Check sheet for the modelled part. Datum: model origin and axes. Units: mm. Give positions to 0.01 mm unless a question says otherwise; leave off trailing zeros. Loops run counter-clockwise (first coordinate to the right, second up) from the corner with the lowest first, then second, coordinate; pieces in that order, holes last. Notation, with made-up numbers: (18.25, -3.75) -> (58.25, -3.75) arc R20 ccw to (58.25, 32.25) -> close; hole circle Ø7 at (65, -7.5). An arc over 180 degrees is marked (long way). Answer as CSV lines item,"result". Start each with the question number.
(1) Section check D-D on z = 2. Enter the section's corners in (x, y), plus the area to 3 significant figures.
(2) Section check B-B on z = 0. Enter the section's corners in (x, y), plus the area to 3 significant figures.
(3) Section check A-A on x = 0. Enter the section's corners in (y, z), plus the area to 3 significant figures.
(4) Material ranges on line 1 (Y direction, x = 0, z = -0.15); line 2 (X direction, y = 14.5, z = 0.45); line 3 (X direction, y = 14.5, z = 0.8), recorded low to high. Write a range as from..to.
(5) Section check C-C on y = 11.75. Enter the section's corners in (x, z).
(6) Release check for a two-part mould opening along X. For faces 1 (the face through (2.385, 9.86, -0.751)), 2 (the face through (-0.098, 15.244, 0.035)), 3 (the face through (0, 0, 0)) record: pulls with the +X half, pulls with the -X half, needs draft (parallel to the pull), parting line crosses it, or undercut.
(7) Gauge pin test, flat ends, axial feed: pin 1 Ø1.5 at (y, z) = (9.5, 1) entering from -X; pin 2 Ø1 at (y, z) = (11.5, -1) entering from -X. Record the tip position at first contact, or that the pin passes through.
from build123d import *

# Parameters (mm, degrees)
CROQUIS1_R                        = 2.5
SALIENTE_EXTRUIR1_DEPTH           = 20
CORTAR_EXTRUIR1_REACH             = 4.5
CROQUIS2_R                        = 0.75
CORTAR_EXTRUIR1_DIRECTION_2_REACH = 4.5


with BuildPart() as part:
    # Croquis1 → Saliente-Extruir1 (new body)
    with BuildSketch(Plane(origin=(0, 0, 0), x_dir=(1, 0, 0), z_dir=(0, 1, 0))):
        Circle(CROQUIS1_R)
    extrude(amount=SALIENTE_EXTRUIR1_DEPTH)

    # Croquis2 → Cortar-Extruir1 (cut, up to next)
    with BuildSketch(Plane.XY, mode=Mode.PRIVATE) as cortar_extruir1_sk1:
        with Locations((0, 14.5)):
            Circle(CROQUIS2_R)
    cortar_extruir1_tool1 = extrude(cortar_extruir1_sk1.sketch, amount=-CORTAR_EXTRUIR1_REACH, mode=Mode.PRIVATE) & part.part
    add(cortar_extruir1_tool1.solids().sort_by_distance((0, 14.5, 0))[0], mode=Mode.SUBTRACT)

    # Croquis2 → Cortar-Extruir1 direction 2 (cut, up to next)
    with BuildSketch(Plane.XY, mode=Mode.PRIVATE) as cortar_extruir1_direction_2_sk1:
        with Locations((0, 14.5)):
            Circle(CROQUIS2_R)
    cortar_extruir1_direction_2_tool1 = extrude(cortar_extruir1_direction_2_sk1.sketch, amount=CORTAR_EXTRUIR1_DIRECTION_2_REACH, mode=Mode.PRIVATE) & part.part
    add(cortar_extruir1_direction_2_tool1.solids().sort_by_distance((0, 14.5, 0))[0], mode=Mode.SUBTRACT)


solid = part.part
Working result:
1,outline,"(-1.5, 0) -> (1.5, 0) -> (1.5, 20) -> (-1.5, 20) -> close; hole circle Ø1.5 at (0, 14.5)"
1,area,"58.2 mm^2"
2,outline,"(-2.5, 0) -> (2.5, 0) -> (2.5, 20) -> (-2.5, 20) -> close; hole circle Ø1.5 at (0, 14.5)"
2,area,"98.2 mm^2"
3,outline,"(0, -2.5) -> (13.75, -2.5) -> (13.75, 2.5) -> (0, 2.5) -> close; (15.25, -2.5) -> (20, -2.5) -> (20, 2.5) -> (15.25, 2.5) -> close"
3,area,"92.5 mm^2"
4,line 1,"y = 0..13.75, 15.25..20"
4,line 2,"x = -2.46..-0.75, 0.75..2.46"
4,line 3,"x = -2.37..-0.75, 0.75..2.37"
5,outline,"circle Ø5 at (0, 0)"
6,face 1,"parting line crosses it"
6,face 2,"undercut"
6,face 3,"needs draft"
7,pin 1,"stops at x = -2.49"
7,pin 2,"stops at x = -2.45"
